Input: part model. Units: mm. Frame: model coordinates. Face numbers are marked on the shaded views. Coordinates: 2 decimals unless noted, no trailing zeros. Loops run counter-clockwise (first coordinate to the right, second up) from the corner with the lowest first, then second, coordinate; pieces in that order, holes last. Notation, with made-up numbers: (65.5, -10.75) -> (117.5, -10.75) arc R25 ccw to (117.5, 18.25) -> close; hole circle Ø6 at (19, 31.5). An arc over 180 degrees is marked (long way). Answer as a JSON object with one key per item and string values.
from build123d import *

# Parameters (mm, degrees)
BASE_FLANGE1_DEPTH = 76.2
SKETCH2_R          = 2.4892
CUT_EXTRUDE1_DEPTH = 83.876344995


# Sheet-metal steps are written as plain solids
with BuildPart() as part:
    # Sketch1 → Base-Flange1 (new body)
    with BuildSketch(Plane.XY):
        with BuildLine():
            Line((-15.00632, -12.7), (-15.00632, -2.4003))
            ThreePointArc((-15.00632, -2.4003), (-14.303288407, -0.703031593), (-12.60602, 0))
            Line((-12.60602, 0), (12.60602, 0))
            ThreePointArc((12.60602, 0), (14.303288407, -0.703031593), (15.00632, -2.4003))
            Line((15.00632, -2.4003), (15.00632, -12.7))
            Line((15.00632, -12.7), (13.41882, -12.7))
            Line((13.41882, -12.7), (13.41882, -2.4003))
            ThreePointArc((13.41882, -2.4003), (13.180756392, -1.825563608), (12.60602, -1.5875))
            Line((12.60602, -1.5875), (-12.60602, -1.5875))
            ThreePointArc((-12.60602, -1.5875), (-13.180756392, -1.825563608), (-13.41882, -2.4003))
            Line((-13.41882, -2.4003), (-13.41882, -12.7))
            Line((-13.41882, -12.7), (-15.00632, -12.7))
        make_face()
    extrude(amount=BASE_FLANGE1_DEPTH)

    # Sketch2 → Cut-Extrude1 (cut, through all)
    with BuildSketch(Plane(origin=(15.00632, 0, 0), x_dir=(0, 0, -1), z_dir=(1, 0, 0))):
        with Locations((-63.5, -7.62)):
            Circle(SKETCH2_R)
        with Locations((-12.7, -7.62)):
            Circle(SKETCH2_R)
    extrude(amount=-CUT_EXTRUDE1_DEPTH, mode=Mode.SUBTRACT)


solid = part.part
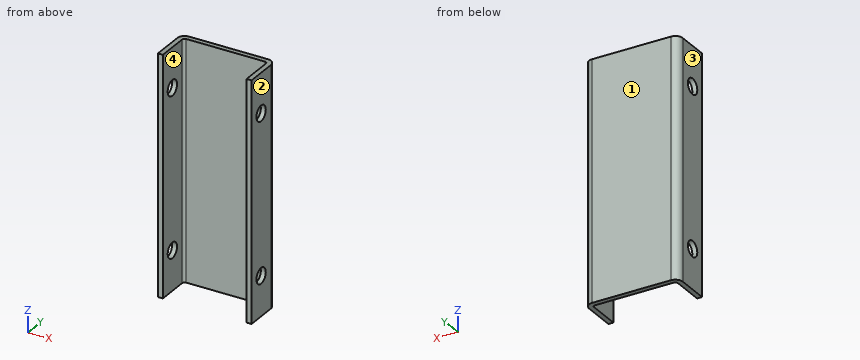
1. Section query B-B (z = 63.5). Return loops of the section in (x, y), plus the area to 3 significant figures.
Reply:
{"outline": "(-15.01, -12.7) -> (-13.42, -12.7) -> (-13.42, -10.11) -> (-15.01, -10.11) -> close; (-15.01, -5.13) -> (-13.42, -5.13) -> (-13.42, -2.4) arc R0.81 cw to (-12.61, -1.59) -> (12.61, -1.59) arc R0.81 cw to (13.42, -2.4) -> (13.42, -5.13) -> (15.01, -5.13) -> (15.01, -2.4) arc R2.4 ccw to (12.61, 0) -> (-12.61, 0) arc R2.4 ccw to (-15.01, -2.4) -> close; (13.42, -12.7) -> (15.01, -12.7) -> (15.01, -10.11) -> (13.42, -10.11) -> close", "area": "64.9 mm2"}
2. Section query D-D (z = 5). Return loops of the section in (x, y).
Reply:
{"outline": "(-15.01, -12.7) -> (-13.42, -12.7) -> (-13.42, -2.4) arc R0.81 cw to (-12.61, -1.59) -> (12.61, -1.59) arc R0.81 cw to (13.42, -2.4) -> (13.42, -12.7) -> (15.01, -12.7) -> (15.01, -2.4) arc R2.4 ccw to (12.61, 0) -> (-12.61, 0) arc R2.4 ccw to (-15.01, -2.4) -> close"}
3. Mould query, pull axis X, two halves, no side actions, for the marked faces 1, 2, 3 and 4. Classes: pulls with the +X half, pulls with the -X half, needs draft (parallel to the pull), parting line crosses it, or undercut.
Reply:
{"face 1": "needs draft", "face 2": "pulls with the +X half", "face 3": "pulls with the -X half", "face 4": "undercut"}
4. Section query A-A (y = -11). Return loops of the section in (x, z), plus the area to 3 significant figures.
Reply:
{"outline": "(-15.01, 0) -> (-13.42, 0) -> (-13.42, 76.2) -> (-15.01, 76.2) -> close; (13.42, 0) -> (15.01, 0) -> (15.01, 76.2) -> (13.42, 76.2) -> close", "area": "242 mm2"}
5. Line query: line 1 along Z through (x, y) = (13.5, -7.5); line 2 along X through (y, z) = (-5, 41); line 3 along X through (y, z) = (-1.75, 4.5). Output: solid intervals per line, ascending.
Reply:
{"line 1": "z = 0 to 10.21, 15.19 to 61.01, 65.99 to 76.2", "line 2": "x = -15.01 to -13.42, 13.42 to 15.01", "line 3": "x = -14.92 to -13.09, 13.09 to 14.92"}
6. Section query C-C (y = -7.62). Return loops of the section in (x, z), plus the area to 3 significant figures.
Reply:
{"outline": "(-15.01, 0) -> (-13.42, 0) -> (-13.42, 10.21) -> (-15.01, 10.21) -> close; (-15.01, 15.19) -> (-13.42, 15.19) -> (-13.42, 61.01) -> (-15.01, 61.01) -> close; (-15.01, 65.99) -> (-13.42, 65.99) -> (-13.42, 76.2) -> (-15.01, 76.2) -> close; (13.42, 0) -> (15.01, 0) -> (15.01, 10.21) -> (13.42, 10.21) -> close; (13.42, 15.19) -> (15.01, 15.19) -> (15.01, 61.01) -> (13.42, 61.01) -> close; (13.42, 65.99) -> (15.01, 65.99) -> (15.01, 76.2) -> (13.42, 76.2) -> close", "area": "210 mm2"}
